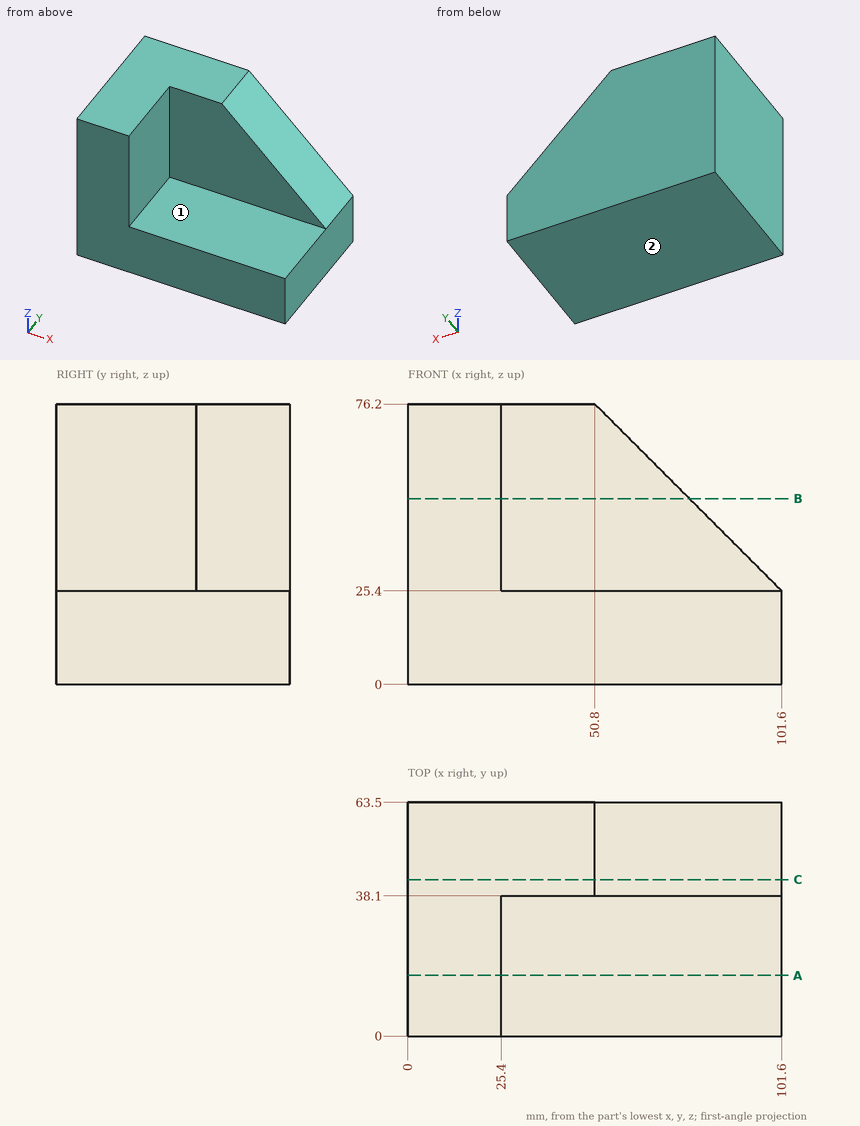
Here's the drawing with two shaded views (mm, measured from the low corner). I have some questions. A direction names the side the tool comes from. Round coordinates to 2 decimals unless told otherwise and drop trailing zeros. Write each loop counter-clockwise with the first axis right and the second up, starting at its lowest first coordinate (ties: lowest second). Pieces come first, ordered by that corner, then holes. Notation, with made-up numbers: M 65.5,75.5 L 70.5,75.5 A17 ccw 70.5,82.5 Z; hole C 11,-36 d5. An arc over 180 degrees is marked long. Write each question's results on one line, items separated by ' | '. Start each with the question number.
1. I need wall thicknesses on L1, parallel to X at y = 18, z = 57; L2, parallel to Y at x = 61.5, z = 44. Which ranges of each line are inside material? Lowest first, please. Write a range as from..to.
2. I'm going to push flat-ended pins straight in: pin 1 Ø11.5 at (y, z) = (22.5, 61.5) entering from +X; pin 2 Ø10 at (x, z) = (59, 65.5) entering from -Y; pin 3 Ø3 at (x, y) = (29.5, 27) entering from +Z. Where does each tip first touch, or does it pass through?
3. Imagine slicing it at B-B on z = 50.5. List the corners of the cut face in (x, y) for me.
4. Imagine slicing it at A-A on y = 16.5. List the corners of the cut face in (x, z) for me.
5. On a 3-axis mill with a long thin cutter (end or side, diameter ignored), from which of +Z, -Z, +X, -X, +Y, -Y can I reach the whole of each face in a straight line? I mean the marked faces 1 and 2. Say none if no direction works.
6. Imagine slicing it at C-C on y = 42.5. List the corners of the cut face in (x, z) for me.
Result sheet:
1) L1: x = 0..25.4 | L2: y = 38.1..63.5
2) pin 1: stops at x = 25.4 | pin 2: stops at y = 38.1 | pin 3: stops at z = 25.4
3) outline: M 0,0 L 25.4,0 L 25.4,38.1 L 76.5,38.1 L 76.5,63.5 L 0,63.5 Z
4) outline: M 0,0 L 101.6,0 L 101.6,25.4 L 25.4,25.4 L 25.4,76.2 L 0,76.2 Z
5) face 1: +Z, +X, -Y | face 2: -Z, +X, -X, +Y, -Y
6) outline: M 0,0 L 101.6,0 L 101.6,25.4 L 50.8,76.2 L 0,76.2 Z
